Could you check a few things on this model? Use its own coordinates, in mm. A direction names the side the tool comes from. Give positions to 0.01 mm unless a question says otherwise; leave off trailing zeros. Loops run counter-clockwise (first coordinate to the right, second up) from the corner with the lowest first, then second, coordinate; pieces in that order, holes last. Notation, with made-up numbers: (-40, 37.5) - (-20, 37.5) arc R9 cw to (-20, 46.5) - close; hole circle Ø10 at (69.5, -32.5). An arc over 180 degrees is marked (long way). Write each question's results on one line, items separated by ' | '. Start each with the question number.
1) If we mould it in two halves opening along Z, with no side actions, what happens to faces 3 (the face through (394, 180, -5)), 4 (the face through (394, 173, 0)), 5 (the face through (800, 173, -394))? For each: +Z half, -Z half, draft (parallel to the pull), parting line (faces both ways), or undercut.
2) I want a section at B-B, the plane z = -580. Write out the boundary of the cut face in (x, y).
3) If I drill on probe 1 along X at (y, z) = (144.5, -198.5); probe 2 along Z at (x, y) = (140.5, 286.5); probe 3 along Y at (x, z) = (155, -171), over which ranges is the centre line in solid material (lowest first)? Write a range as [from, to].
4) I'm going to push a flat-ended pin straight in: pin 1 (1.5 mm diameter, centred on x = 185.5, z = -513.5, fed in from +Y). Where does the tip first touch, or does it pass through?
5) I want a section at A-A, the plane y = 203. Write out the boundary of the cut face in (x, z), and give its area (3 significant figures).
6) On a 3-axis mill with a long thin cutter (end or side, diameter ignored), from which of +Z, -Z, +X, -X, +Y, -Y can I reach the whole of each face in a straight line? I mean faces 1 (the face through (394, 180, -795)), 2 (the face through (394, 0, -406)). Say none if no direction works.
7) I want a section at D-D, the plane x = 398.5. Write out the boundary of the cut face in (y, z).
8) I want a section at C-C, the plane z = -140. Write out the boundary of the cut face in (x, y), and give its area (3 significant figures).
from build123d import *

# Parameters (mm, degrees)
SKIZZE1_W                            = 800
SKIZZE1_H                            = 800
AUFSATZ_LINEAR_AUSTRAGEN1_DEPTH      = 350
SKIZZE2_W                            = 790
SKIZZE2_H                            = 790
SCHNITT_LINEAR_AUSTRAGEN1_DEPTH      = 345
SCHNITT_LINEAR_AUSTRAGEN2_DEPTH      = 1185.271928233
SCHNITT_LINEAR_AUSTRAGEN2_DEPTH_BACK = 1185.271928233


with BuildPart() as part:
    # Skizze1 → Aufsatz-Linear austragen1 (new body)
    with BuildSketch(Plane(origin=(0, 0, 0), x_dir=(1, 0, 0), z_dir=(0, 1, 0))):
        with Locations((400, 400)):
            Rectangle(SKIZZE1_W, SKIZZE1_H)
    extrude(amount=AUFSATZ_LINEAR_AUSTRAGEN1_DEPTH)

    # Skizze2 → Schnitt-Linear austragen1 (cut)
    with BuildSketch(Plane(origin=(0, 350, 0), x_dir=(1, 0, 0), z_dir=(0, 1, 0))):
        with Locations((400, 400)):
            Rectangle(SKIZZE2_W, SKIZZE2_H)
    extrude(amount=-SCHNITT_LINEAR_AUSTRAGEN1_DEPTH, mode=Mode.SUBTRACT)

    # Skizze3 → Schnitt-Linear austragen2 (cut, two sides: drawn at the far end of the back side and taken through both)
    with BuildSketch(Plane(origin=(800, 0, 0), x_dir=(0, 0, -1), z_dir=(1, 0, 0)).offset(-SCHNITT_LINEAR_AUSTRAGEN2_DEPTH_BACK)):
        with BuildLine():
            Line((210, 300), (590, 300))
            ThreePointArc((590, 300), (597.071067812, 297.071067812), (600, 290))
            Line((600, 290), (600, 260))
            ThreePointArc((600, 260), (597.071067812, 252.928932188), (590, 250))
            Line((590, 250), (210, 250))
            ThreePointArc((210, 250), (202.928932188, 252.928932188), (200, 260))
            Line((200, 260), (200, 290))
            ThreePointArc((200, 290), (202.928932188, 297.071067812), (210, 300))
        make_face()
    extrude(amount=SCHNITT_LINEAR_AUSTRAGEN2_DEPTH + SCHNITT_LINEAR_AUSTRAGEN2_DEPTH_BACK, mode=Mode.SUBTRACT)


solid = part.part
Answers:
1) face 3: undercut | face 4: +Z half | face 5: draft
2) outline: (0, 0) - (800, 0) - (800, 250) - (795, 250) - (795, 5) - (5, 5) - (5, 250) - (0, 250) - close; (0, 300) - (5, 300) - (5, 350) - (0, 350) - close; (795, 300) - (800, 300) - (800, 350) - (795, 350) - close
3) probe 1: x = [0, 5], [795, 800] | probe 2: z = [-800, -795], [-5, 0] | probe 3: y = [0, 5]
4) pin 1: stops at y = 5
5) outline: (0, -800) - (800, -800) - (800, 0) - (0, 0) - close; hole (5, -795) - (795, -795) - (795, -5) - (5, -5) - close | area: 15,900 mm2
6) face 1: +Y | face 2: +Z, -Z, +X, -X, -Y
7) outline: (0, -800) - (350, -800) - (350, -795) - (5, -795) - (5, -5) - (350, -5) - (350, 0) - (0, 0) - close
8) outline: (0, 0) - (800, 0) - (800, 350) - (795, 350) - (795, 5) - (5, 5) - (5, 350) - (0, 350) - close | area: 7,450 mm2
